Autodesk Inventor part; units mm, degrees
ref_plane "Work Plane1" through (0, 0, 10.7) normal (0, 0, 1) x (1, 0, 0)
ref_plane "YZ Plane" through (0, 0, 0) normal (1, 0, 0) x (0, 1, 0)
ref_plane "XZ Plane" through (0, 0, 0) normal (0, 1, 0) x (-1, 0, 0)
sketch "Sketch1" plane through (0, 0, 0) normal (0, 0, 1) x (1, 0, 0)
  line L0 (-8, -2) -> (8, -2)
  line L1 (8, -2) -> (8, 2)
  line L2 (8, 2) -> (-8, 2)
  line L3 (-8, 2) -> (-8, -2)
  point P0 (0, 0)
  dimension "d268" = 4
  dimension "d269" = 2
  dimension "d270" = 16
  dimension "d271" = 8
extrude "Extrusion1" add sketch "Sketch1" along normal blind 10.2
sketch "Sketch2" plane through (-6.98, -2.75, 0) normal (0, -1, 0) x (1, 0, 0)
  line L0 (0, 0) -> (13.96, 0)
  line L1 (5.18, 3.6) -> (8.78, 3.6)
  line L2 (8.78, 3.6) -> (8.78, 0.5)
  line L3 (8.28, 0) -> (5.68, 0)
  line L4 (5.18, 0.5) -> (5.18, 3.6)
  line L5 (5.18, 0.5) -> (5.68, 0)
  line L6 (8.78, 0.5) -> (8.28, 0)
  point P0 (6.98, 0)
  dimension "d15" = 3.6
  dimension "d17" = 0.5
  dimension "d19" = 135
  dimension "d20" = 135
  dimension "d21" = 0.5
  dimension "d22" = 3.6
extrude "Extrusion2" [suppressed]
sketch "Sketch3" plane through (0, 0, 0) normal (0, 1, 0) x (-1, 0, 0)
  line L0 (-6.98, 3.6) -> (-7.23, 3.6)
  line L1 (-7.98, 2.1) -> (-7.98, 1.22)
  line L2 (-7.98, 1.22) -> (-6.98, 1.22)
  line L3 (-6.98, 1.22) -> (-6.98, 3.6)
  line L4 (6.98, 10.2) -> (-6.98, 10.2)
  line L5 (0, 10.2) -> (0, 0)
  line L6 (-6.98, 0) -> (6.98, 0)
  line L7 (-7.23, 3.6) -> (-7.98, 2.1)
  line L8 (6.98, 3.6) -> (7.23, 3.6)
  line L9 (7.98, 2.1) -> (7.98, 1.22)
  line L10 (7.98, 1.22) -> (6.98, 1.22)
  line L11 (6.98, 1.22) -> (6.98, 3.6)
  line L12 (7.23, 3.6) -> (7.98, 2.1)
  dimension "d25" = 13.96
  dimension "d26" = 1.22
  dimension "d28" = 1
  dimension "d29" = 1.5
  dimension "d30" = 0.88
  dimension "d31" = 0.25
extrude "Extrusion3" [suppressed]
sketch "Sketch4" plane through (0, -0.5, 0) normal (0, -1, 0) x (1, 0, 0)
  line L0 (6.98, 3.6) -> (7.23, 3.6)
  line L1 (6.98, 6.263) -> (7.23, 6.263)
  line L2 (7.98, 5.513) -> (7.98, 5.263)
  line L3 (7.98, 5.263) -> (6.98, 5.263)
  line L4 (6.98, 5.263) -> (6.98, 6.263)
  line L5 (-6.98, 10.2) -> (6.98, 10.2)
  line L6 (6.98, 0) -> (-6.98, 0)
  line L7 (0, 10.2) -> (0, 0)
  line L8 (7.23, 6.263) -> (7.98, 5.513)
  line L9 (-6.98, 6.263) -> (-7.23, 6.263)
  line L10 (-7.98, 5.513) -> (-7.98, 5.263)
  line L11 (-7.98, 5.263) -> (-6.98, 5.263)
  line L12 (-6.98, 5.263) -> (-6.98, 6.263)
  line L13 (-7.23, 6.263) -> (-7.98, 5.513)
  dimension "d34" = 1.663
  dimension "d35" = 13.96
  dimension "d36" = 1
  dimension "d38" = 0.25
  dimension "d39" = 1
  dimension "d40" = 0.25
extrude "Extrusion4" [suppressed]
sketch "Sketch5" plane through (0, 0.5, 0) normal (0, 1, 0) x (1, 0, 0)
  line L0 (7.23, -3.6) -> (6.98, -3.6)
  line L1 (7.23, -6.263) -> (6.98, -6.263)
  line L2 (6.98, -6.263) -> (6.98, -5.263)
  line L3 (6.98, -5.263) -> (7.98, -5.263)
  line L4 (7.98, -5.263) -> (7.98, -5.513)
  line L5 (6.98, -10.2) -> (-6.98, -10.2)
  line L6 (1.3, 0) -> (-1.3, 0)
  line L7 (0, 0) -> (0, -10.2)
  line L8 (7.23, -6.263) -> (7.98, -5.513)
  line L9 (-7.23, -6.263) -> (-6.98, -6.263)
  line L10 (-6.98, -6.263) -> (-6.98, -5.263)
  line L11 (-6.98, -5.263) -> (-7.98, -5.263)
  line L12 (-7.98, -5.263) -> (-7.98, -5.513)
  line L13 (-7.23, -6.263) -> (-7.98, -5.513)
  dimension "d43" = 1.663
  dimension "d44" = 13.96
  dimension "d45" = 1
  dimension "d46" = 1
  dimension "d47" = 0.25
  dimension "d48" = 0.25
extrude "Extrusion5" [suppressed]
sketch "Sketch6" plane through (-6.98, -2.75, 10.2) normal (0, -1, 0) x (1, 0, 0)
  line L0 (0, -10.2) -> (5.68, -10.2)
  line L1 (-38.97, -10.2) -> (-36.97, -6.7359)
  line L2 (-36.97, -6.7359) -> (-34.97, -10.2)
  line L3 (-38.97, -10.2) -> (-34.97, -10.2)
  line L4 (0.5, -10.2) -> (2.5, -6.7359)
  line L5 (2.5, -6.7359) -> (4.5, -10.2)
  line L6 (0.5, -10.2) -> (4.5, -10.2)
  dimension "d61" = 0.5
  dimension "d62" = 4
extrude "Extrusion6" [suppressed]
sketch "Sketch7" plane through (0, 0, 0) normal (0, 0, -1) x (-1, 0, 0)
  line L0 (6.98, 2.75) -> (6.98, -1.25)
  line L1 (4.705, 1.645) -> (5.455, 1.645)
  line L2 (5.455, 1.645) -> (5.455, 0.895)
  line L3 (5.455, 0.895) -> (4.705, 0.895)
  line L4 (4.705, 0.895) -> (4.705, 1.645)
  line L5 (4.705, -0.895) -> (5.455, -0.895)
  line L6 (5.455, -0.895) -> (5.455, -1.645)
  line L7 (5.455, -1.645) -> (4.705, -1.645)
  line L8 (4.705, -1.645) -> (4.705, -0.895)
  line L9 (5.08, 0.895) -> (5.08, -0.895) construction
  point P0 (0, 0)
  point P1 (5.08, 0)
  dimension "d65" = 0.75
  dimension "d66" = 2.54
  dimension "d67" = 1.525
extrude "Extrusion7" [suppressed]
chamfer "Chamfer1" [suppressed]
pattern_linear "Rectangular Pattern1" [suppressed]
ref_plane "Work Plane1" through (0, 0, 10.7) normal (0, 0, 1) x (1, 0, 0)
sketch "Sketch8" plane through (0, 0, 10.7) normal (0, 0, 1) x (1, 0, 0)
  line L0 (-6.98, 2.75) -> (6.98, 2.75)
  line L1 (-6.98, -2.75) -> (-6.98, 2.75)
  line L2 (6.98, -2.75) -> (-6.98, -2.75)
  line L3 (6.98, 2.75) -> (6.98, -2.75)
  line L4 (-7.11, 0) -> (-42.9538, 0)
  line L5 (-8, -2) -> (-8, 2)
  line L6 (8, -2) -> (-8, -2)
  line L7 (8, 2) -> (8, -2)
  line L8 (-8, 2) -> (8, 2)
  line L9 (8, 2) -> (-8, 2)
  line L10 (8, -2) -> (-8, -2)
  line L11 (-8, -2) -> (-8, 2)
  line L12 (-8, 2) -> (8, 2)
  line L13 (8, 2) -> (8, -2)
extrude "Extrusion20" add sketch "Sketch8" along normal blind 0.8 contours L8 L3 L6 L1 | L1 L6 L5 L8 | L8 L7 L6 L3
sketch "Sketch22" plane through (0, 0, 0) normal (0, 0, -1) x (-1, 0, 0)
  line L0 (-7.99, -3) -> (-8.665, -3)
  line L1 (8.665, 2.75) -> (-8.665, 2.75)
  line L2 (-8.665, -3) -> (8.665, -3)
  line L3 (8.665, -3) -> (8.665, 2.75)
  line L4 (8.665, 2.75) -> (-8.665, 2.75)
  line L5 (-8.665, 2.75) -> (-8.665, -3)
  point P0 (0, 0)
extrude "Extrusion17" [suppressed]
sketch "Sketch25" plane through (0, 0, 0) normal (0, 0, -1) x (-1, 0, 0)
  line L0 (8, -2) -> (-8, -2)
  line L1 (8, 2) -> (8, -2)
  line L2 (-8, 2) -> (8, 2)
  line L3 (-8, -2) -> (-8, 2)
  line L4 (8, -2) -> (-8, -2)
  line L5 (-8, -2) -> (-8, 2)
  line L6 (-8, 2) -> (8, 2)
  line L7 (8, 2) -> (8, -2)
  point P0 (0, 0)
extrude "Extrusion21" cut sketch "Sketch25" against normal blind 9.1
sketch "Sketch26" plane through (0, 0, 10.2) normal (0, 0, 1) x (1, 0, 0)
  line L0 (8, -2) -> (-8, -2)
  line L1 (8, 2) -> (-8, 2)
  line L2 (-8, -2) -> (-7, -2)
  line L3 (-7, -2) -> (-7, 2)
  line L4 (-7, 2) -> (-8, 2)
  line L5 (-8, 2) -> (-8, -2)
  point P0 (0, 0)
  dimension "d276" = 1
extrude "Extrusion22" add sketch "Sketch26" along normal blind 0.5
mirror "Mirror1" about plane through (0, 0, 0) normal (1, 0, 0) of "Extrusion22"
equation "\"DimA\" = 13.96"
equation "\"DimB\" = 17.33"
equation "\"DimC\" = 5.715"
properties part number "Ribbon Cable Connector-02"
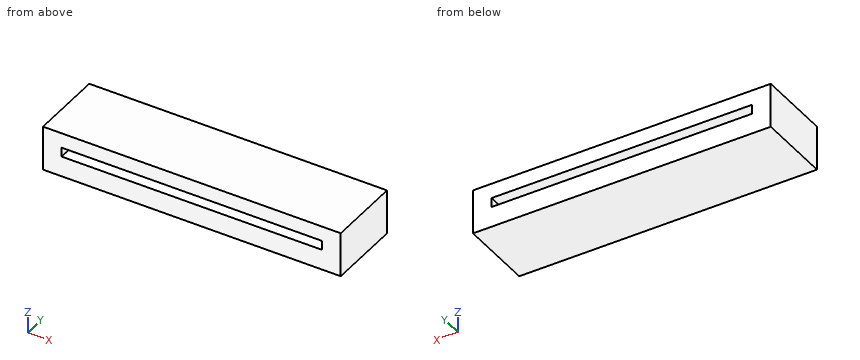
CAD build for the part. Positions are in the model's coordinates, mm. Coordinates: 2 decimals unless noted, no trailing zeros. Loops run counter-clockwise (first coordinate to the right, second up) from the corner with the lowest first, then second, coordinate; pieces in that order, holes last. Notation, with made-up numbers: (46.25, 27.25) - (79.25, 27.25) arc R30 cw to (79.25, 49.25) - close; hole circle Ø1 at (17, -19). An arc over 180 degrees is marked (long way). Use CSV: the item, a comma, the result in double quotes. Start each with the question number.
Q1. Cut at B-B, the plane z = 10.5. List the corners of the cut face in (x, y).
Q2. Cut at C-C, the plane y = 0.9. List the corners of the cut face in (x, z), then the cut area to 3 significant figures.
Q3. Cut at A-A, the plane x = -4.25. List the corners of the cut face in (y, z), then the cut area to 3 significant figures.
Q4. Probe probe 1 along X at (y, z) = (0.85, 10.25); probe 2 along Z at (x, y) = (-3.25, 0.3). List the from-to ranges inside material, lowest first. Write a range as from..to.
Here are the results:
1,outline,"(-8, -2) - (-7, -2) - (-7, 2) - (-8, 2) - close; (7, -2) - (8, -2) - (8, 2) - (7, 2) - close"
2,outline,"(-8, 9.1) - (8, 9.1) - (8, 11.5) - (-8, 11.5) - close; hole (-7, 10.2) - (7, 10.2) - (7, 10.7) - (-7, 10.7) - close"
2,area,"31.4 mm2"
3,outline,"(-2, 9.1) - (2, 9.1) - (2, 10.2) - (-2, 10.2) - close; (-2, 10.7) - (2, 10.7) - (2, 11.5) - (-2, 11.5) - close"
3,area,"7.60 mm2"
4,probe 1,"-8..-7, 7..8"
4,probe 2,"9.1..10.2, 10.7..11.5"
